Job drawing, mm, ordinate dimensions from the low corner. One solid piece. A direction names the side the tool comes from. Coordinates: 2 decimals unless noted, no trailing zeros. Write each loop counter-clockwise with the first axis right and the second up, starting at its lowest first coordinate (ties: lowest second). Pieces come first, ordered by that corner, then holes.
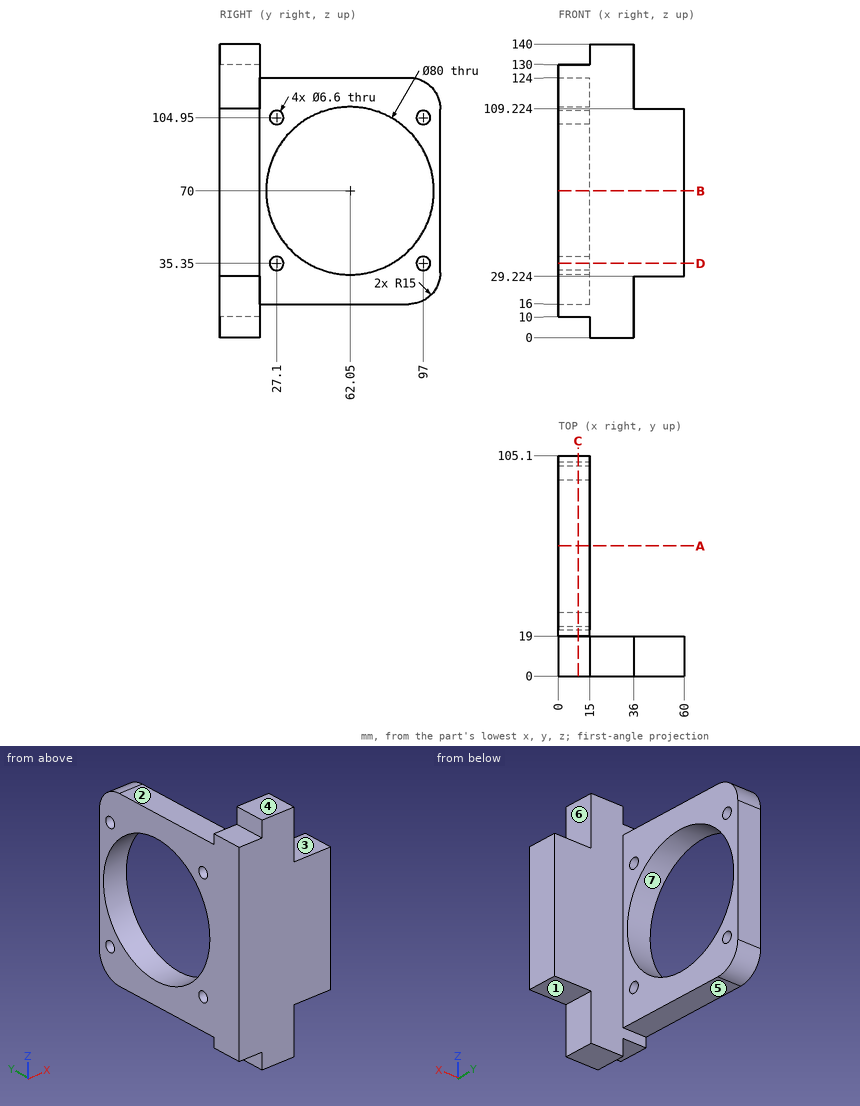
1. 3-axis set-ups, long thin cutter, end or side, ignore diameter. For the marked faces 1, 2 and 3: which of +Z, -Z, +X, -X, +Y, -Y reach the whole face in a straight line?
Computed values:
face 1: -Z, +X, +Y, -Y
face 2: +Z, +X, -X, +Y
face 3: +Z, +X, +Y, -Y
2. Saw through at A-A on y = 62.05. List the corners of the cut face in (x, z).
Computed values:
outline: (0, 16) - (15, 16) - (15, 30) - (0, 30) - close; (0, 110) - (15, 110) - (15, 124) - (0, 124) - close
3. Probe line 1 along Y through (x, z) = (3, 35.35) (1 decimal); line 2 along Y through (x, z) = (17.5, 96.5); line 3 along Y through (x, z) = (11.5, 70). List the from-to ranges inside material, lowest first.
Computed values:
line 1: y = 0 to 23.8, 30.4 to 42.1, 82 to 93.7, 100.3 to 105.1
line 2: y = 0 to 19
line 3: y = 0 to 22.05, 102.05 to 105.1
4. Mould opens along Z. For the marked faces 4, 5, 6 and 7 say: +Z half, -Z half, draft (parallel to the pull), parting line (faces both ways), or undercut.
Computed values:
face 4: +Z half
face 5: -Z half
face 6: draft
face 7: undercut
5. Saw through at B-B on z = 70. List the corners of the cut face in (x, y), plus the area to 3 significant figures.
Computed values:
outline: (0, 0) - (60, 0) - (60, 19) - (15, 19) - (15, 22.05) - (0, 22.05) - close; (0, 102.05) - (15, 102.05) - (15, 105.1) - (0, 105.1) - close
area: 1,230 mm2
6. Saw through at D-D on z = 35.35. List the corners of the cut face in (x, y) (1 decimal).
Computed values:
outline: (0, 0) - (60, 0) - (60, 19) - (15, 19) - (15, 23.8) - (0, 23.8) - close; (0, 30.4) - (15, 30.4) - (15, 42.1) - (0, 42.1) - close; (0, 82) - (15, 82) - (15, 93.7) - (0, 93.7) - close; (0, 100.3) - (15, 100.3) - (15, 105.1) - (0, 105.1) - close
7. Saw through at C-C on x = 9.5. List the corners of the cut face in (y, z).
Computed values:
outline: (0, 10) - (19, 10) - (19, 16) - (90.1, 16) arc R15 ccw to (105.1, 31) - (105.1, 109) arc R15 ccw to (90.1, 124) - (19, 124) - (19, 130) - (0, 130) - close; hole circle Ø80 at (62.05, 70); hole circle Ø6.6 at (27.1, 35.35); hole circle Ø6.6 at (27.1, 104.95); hole circle Ø6.6 at (97, 35.35); hole circle Ø6.6 at (97, 104.95)
8. Flat gauge pins, fed straight in: pin 1 (7.5 mm diameter, centred on y = 97, z = 104.95, fed in from -X); pin 2 (12 mm diameter, centred on x = 32.5, z = 58, fed in from +Y); pin 3 (4.5 mm diameter, centred on x = 5, y = 6, fed in from -Z); pin 4 (9.5 mm diameter, centred on y = 5, z = 117, fed in from +X). Where does each tip first touch, or does it go through?
Computed values:
pin 1: stops at x = 0
pin 2: stops at y = 19
pin 3: stops at z = 10
pin 4: stops at x = 36
